from build123d import *

# Parameters (mm, degrees)
SKETCH_1_W              = 48
SKETCH_1_H              = 20
EXTRUDE_1_DEPTH         = 30
SKETCH_2_W              = 14
SKETCH_2_H              = 30
CUT_EXTRUDE_1_DEPTH     = 7
EXTRUDE_2_DEPTH         = 48
CUT_EXTRUDE_2_DEPTH     = 14
CUT_EXTRUDE_3_DEPTH     = 14
CUT_EXTRUDE_4_DEPTH     = 65.456478054
SKETCH_13_R             = 4
CUT_EXTRUDE_5_DEPTH     = 53.52066051
SKETCH_14_R             = 4
CUT_EXTRUDE_6_DEPTH     = 53.52066051
FILLET_1_R              = 7
EXTRUDE_3_DEPTH         = 3
EXTRUDE_5_DEPTH         = 1
SKETCH_20_R             = 7.5
CUT_EXTRUDE_8_DEPTH     = 53.520660579
BOSS_EXTRUDE1_DEPTH     = 25
CUT_EXTRUDE1_DEPTH      = 80.244164279
CUT_EXTRUDE1_DEPTH_BACK = 80.244164279


with BuildPart() as part:
    # Эскиз1 → Бобышка-Вытянуть1 (new body)
    with BuildSketch(Plane(origin=(0, 0, 0), x_dir=(1, 0, 0), z_dir=(0, 1, 0))):
        Rectangle(SKETCH_1_W, SKETCH_1_H)
    extrude(amount=EXTRUDE_1_DEPTH)

    # Эскиз2 → Вырез-Вытянуть1 (cut)
    with BuildSketch(Plane.XY.offset(10)):
        with Locations((0, 15)):
            Rectangle(SKETCH_2_W, SKETCH_2_H)
    extrude(amount=-CUT_EXTRUDE_1_DEPTH, mode=Mode.SUBTRACT)

    # Эскиз7 → Бобышка-Вытянуть2 (add)
    with BuildSketch(Plane(origin=(24, 0, 0), x_dir=(0, 0, -1), z_dir=(1, 0, 0))):
        Polygon((10, 0), (27.320508076, -10), (45.810889132, 22.026279442), (32, 30), (10, 30), align=None)
    extrude(amount=-EXTRUDE_2_DEPTH)

    # Эскиз8 → Вырез-Вытянуть2 (cut)
    with BuildSketch(Plane(origin=(24, 0, 0), x_dir=(0, 0, -1), z_dir=(1, 0, 0))):
        Polygon((10, 0), (10, 30), (32, 30), (45.810889132, 22.026279442), (27.320508076, -10), align=None)
    extrude(amount=-CUT_EXTRUDE_2_DEPTH, mode=Mode.SUBTRACT)

    # Эскиз9 → Вырез-Вытянуть3 (cut)
    with BuildSketch(Plane.ZY.offset(24)):
        Polygon((-10, 0), (-10, 30), (-32, 30), (-45.810889132, 22.026279442), (-27.320508076, -10), align=None)
    extrude(amount=-CUT_EXTRUDE_3_DEPTH, mode=Mode.SUBTRACT)

    # Эскиз11 → Вырез-Вытянуть4 (cut, through all)
    with BuildSketch(Plane.ZY.offset(10)):
        Polygon((-17.085266521, 5.482226936), (-27.285266521, 23.149145173), (-36.291930721, 17.949145173), (-26.091930721, 0.282226936), align=None)
    extrude(amount=-CUT_EXTRUDE_4_DEPTH, mode=Mode.SUBTRACT)

    # Эскиз13 → Вырез-Вытянуть5 (cut, through all)
    with BuildSketch(Plane(origin=(0, 0, -10), x_dir=(-1, 0, 0), z_dir=(0, 0, -1))):
        with Locations((17, 15)):
            Circle(SKETCH_13_R)
    extrude(amount=-CUT_EXTRUDE_5_DEPTH, mode=Mode.SUBTRACT)

    # Эскиз14 → Вырез-Вытянуть6 (cut, through all)
    with BuildSketch(Plane(origin=(0, 0, -10), x_dir=(-1, 0, 0), z_dir=(0, 0, -1))):
        with Locations((-17, 15)):
            Circle(SKETCH_14_R)
    extrude(amount=-CUT_EXTRUDE_6_DEPTH, mode=Mode.SUBTRACT)

    # Скругление1
    fillet_1_edges = [part.edges().sort_by_distance(p)[0] for p in [
        (-7, 15, 3),
        (7, 15, 3),
    ]]
    fillet(fillet_1_edges, radius=FILLET_1_R - 0.0001)  # a hair under: the kernel refuses the full size

    # Эскиз16 → Бобышка-Вытянуть3 (add)
    with BuildSketch(Plane(origin=(10, 0, 0), x_dir=(0, 0, -1), z_dir=(1, 0, 0))):
        Polygon((27.285266521, 23.149145173), (17.085266521, 5.482226936), (26.091930721, 0.282226936), (36.291930721, 17.949145173), align=None)
    extrude(amount=-EXTRUDE_3_DEPTH)

    # Эскиз18 → Бобышка-Вытянуть5 (add)
    with BuildSketch(Plane(origin=(0, -14.330127019, -24.820508076), x_dir=(-1, 0, 0), z_dir=(0, -0.4999999999999885, -0.8660254037844454))):
        with BuildLine():
            Line((3.076923077, 23.490381057), (3.076923077, 15.490381057))
            Line((3.076923077, 15.490381057), (-0.394230769, 15.490381057))
            add(Edge.make_bspline(
                [(-0.394230769, 15.490381057), (-0.475966203, 15.49101845), (-0.634155568, 15.49225205), (-0.863556464, 15.501067061), (-1.077173272, 15.519794557), (-1.276352297, 15.540710881), (-1.460752713, 15.571594241), (-1.630462401, 15.607825992), (-1.784830485, 15.650647709), (-1.925031539, 15.701264755), (-2.055118116, 15.758511595), (-2.175664232, 15.829183977), (-2.291845901, 15.906492451), (-2.399031866, 15.998074814), (-2.502049745, 16.096470161), (-2.596586483, 16.206601733), (-2.685439891, 16.325713037), (-2.793473896, 16.498197991), (-2.906939016, 16.729401784), (-3.004668447, 17.02314385), (-3.06681146, 17.330727068), (-3.073519576, 17.5408315), (-3.076923077, 17.647432339)],
                knots=[0, 0, 0, 0, 1.242075696, 2.40389213, 3.487198984, 4.500157661, 5.446319301, 6.326791195, 7.136300648, 7.878370406, 8.590488565, 9.292260633, 9.999224673, 10.708050372, 11.431369221, 12.162165018, 12.910600795, 13.687589445, 15.252257874, 16.810406251, 18.381693487, 20, 20, 20, 20], degree=3))
            add(Edge.make_bspline(
                [(-3.076923077, 17.647432339), (-3.075357604, 17.715865612), (-3.072265688, 17.851026019), (-3.048581646, 18.049748215), (-3.005726368, 18.239618444), (-2.950775925, 18.42230348), (-2.87555432, 18.595200652), (-2.788453183, 18.761894703), (-2.680395045, 18.917607923), (-2.559742342, 19.067544403), (-2.419445088, 19.204937793), (-2.263386964, 19.331922341), (-2.086876234, 19.440896432), (-1.89570213, 19.542168691), (-1.684937787, 19.625339579), (-1.457761732, 19.698574242), (-1.21241575, 19.755040234), (-1.042362796, 19.783482773), (-0.955128205, 19.798073364)],
                knots=[0, 0, 0, 0, 0.982645791, 1.940792824, 2.867691729, 3.775150443, 4.675643875, 5.571354211, 6.471357401, 7.392684514, 8.331098131, 9.285922955, 10.275520706, 11.304845665, 12.388884831, 13.524255008, 14.729980297, 16, 16, 16, 16], degree=3))
            add(Edge.make_bspline(
                [(-0.955128205, 19.798073364), (-1.019738399, 19.830278555), (-1.14226585, 19.891352818), (-1.308999482, 19.992404668), (-1.455065559, 20.087536339), (-1.53803712, 20.158871679), (-1.576923077, 20.192304134)],
                knots=[0, 0, 0, 0, 1.172551213, 2.223638478, 3.167479604, 4, 4, 4, 4], degree=3))
            add(Edge.make_bspline(
                [(-1.576923077, 20.192304134), (-1.652624383, 20.266285408), (-1.807875296, 20.418008818), (-2.019735444, 20.678834883), (-2.229368535, 20.965668904), (-2.355227865, 21.174690137), (-2.419871795, 21.282047723)],
                knots=[0, 0, 0, 0, 0.918170575, 1.883016652, 2.912673989, 4, 4, 4, 4], degree=3))
            Line((-2.419871795, 21.282047723), (-3.732371795, 23.490381057))
            Line((-3.732371795, 23.490381057), (-2.439102564, 23.490381057))
            Line((-2.439102564, 23.490381057), (-1.442307692, 21.801278493))
            add(Edge.make_bspline(
                [(-1.442307692, 21.801278493), (-1.406465761, 21.74201577), (-1.337009983, 21.627174345), (-1.236719552, 21.459429826), (-1.138255761, 21.30508177), (-1.047376022, 21.15932531), (-0.958316878, 21.02600434), (-0.878481314, 20.900073272), (-0.798305584, 20.788666158), (-0.706246053, 20.654823189), (-0.593818414, 20.510114732), (-0.462623309, 20.361457059), (-0.34199814, 20.238315643), (-0.18956943, 20.120822362), (-3.2323e-05, 20.013245791), (0.159774488, 19.962214344), (0.237179487, 19.937496441)],
                knots=[0, 0, 0, 0, 1.130591283, 2.190900266, 3.190104209, 4.119071823, 4.994606968, 5.807262858, 6.55236009, 7.234593472, 8.459046683, 9.540234366, 10.471327768, 11.266723835, 12.676093724, 14, 14, 14, 14], degree=3))
            add(Edge.make_bspline(
                [(0.237179487, 19.937496441), (0.269697183, 19.931632396), (0.343936058, 19.918244603), (0.469993483, 19.909501015), (0.622727518, 19.900220866), (0.733416476, 19.900491258), (0.793269231, 19.900637467)],
                knots=[0, 0, 0, 0, 0.709978628, 1.620902492, 2.713552433, 4, 4, 4, 4], degree=3))
            Line((0.793269231, 19.900637467), (1.948717949, 19.900637467))
            Line((1.948717949, 19.900637467), (1.948717949, 23.490381057))
            Line((1.948717949, 23.490381057), (3.076923077, 23.490381057))
        make_face()
        with BuildLine():
            Line((1.948717949, 18.977560544), (-0.193910256, 18.977560544))
            add(Edge.make_bspline(
                [(-0.193910256, 18.977560544), (-0.301354607, 18.97589409), (-0.502211742, 18.972778811), (-0.783007271, 18.945769758), (-1.023200158, 18.903550736), (-1.225858519, 18.839427155), (-1.396173113, 18.753553027), (-1.54378517, 18.648537277), (-1.667901131, 18.51825252), (-1.769975791, 18.368861713), (-1.849770319, 18.206056724), (-1.90552669, 18.03374763), (-1.942959563, 17.855238544), (-1.946787014, 17.733092852), (-1.948717949, 17.6714708)],
                knots=[0, 0, 0, 0, 1.546056516, 2.890207646, 4.055830773, 5.050253158, 5.937355789, 6.790906573, 7.644595853, 8.512568064, 9.38593768, 10.244184789, 11.114197691, 12, 12, 12, 12], degree=3))
            add(Edge.make_bspline(
                [(-1.948717949, 17.6714708), (-1.947235583, 17.626563151), (-1.944332064, 17.538602257), (-1.928948857, 17.409542216), (-1.89968097, 17.287236957), (-1.859266003, 17.17080484), (-1.808094758, 17.059993077), (-1.745213393, 16.955237495), (-1.670946372, 16.857073145), (-1.585753391, 16.765016757), (-1.487970747, 16.681241729), (-1.376270424, 16.608965458), (-1.251544399, 16.547545272), (-1.113644587, 16.498798364), (-0.963006292, 16.459808698), (-0.798771701, 16.43387015), (-0.621691971, 16.415101097), (-0.498985984, 16.414015918), (-0.435897436, 16.41345798)],
                knots=[0, 0, 0, 0, 0.965235723, 1.89061323, 2.787065514, 3.661873922, 4.534873316, 5.404925039, 6.281839248, 7.175200054, 8.095223355, 9.040740021, 10.02630299, 11.075573487, 12.177989335, 13.364883635, 14.645170704, 16, 16, 16, 16], degree=3))
            Line((-0.435897436, 16.41345798), (1.948717949, 16.41345798))
            Line((1.948717949, 16.41345798), (1.948717949, 18.977560544))
        make_face(mode=Mode.SUBTRACT)
    extrude(amount=EXTRUDE_5_DEPTH)

    # Эскиз20 → Вырез-Вытянуть8 (cut, through all)
    with BuildSketch(Plane(origin=(0, 0, -10), x_dir=(-1, 0, 0), z_dir=(0, 0, -1))):
        with Locations((-17, 15)):
            Circle(SKETCH_20_R)
        with Locations((17, 15)):
            Circle(SKETCH_20_R)
    extrude(amount=CUT_EXTRUDE_8_DEPTH, mode=Mode.SUBTRACT)

    # Sketch3 → Boss-Extrude1 (add)
    with BuildSketch(Plane(origin=(0, 30, 0), x_dir=(1, 0, 0), z_dir=(0, 1, 0))):
        with BuildLine():
            Line((7, -10), (24, -10))
            Line((24, -10), (24, 10))
            Line((24, 10), (10, 10))
            Line((10, 10), (10, 32))
            Line((10, 32), (-10, 32))
            Line((-10, 32), (-10, 10))
            Line((-10, 10), (-24, 10))
            Line((-24, 10), (-24, -10))
            Line((-24, -10), (-7, -10))
            ThreePointArc((-7, -10), (0, -3), (7, -10))
        make_face()
    extrude(amount=BOSS_EXTRUDE1_DEPTH)

    # Sketch4 → Cut-Extrude1 (cut, two sides: drawn at the far end of the back side and taken through both)
    with BuildSketch(Plane.ZY.offset(10).offset(-CUT_EXTRUDE1_DEPTH_BACK)):
        Polygon((-251.050138586, -96.468656479), (-45.810889132, 22.026279442), (35.63071017, 69.046608722), (240.869959624, 187.541544642), (3.880087783, 598.020043549), (-488.040010426, 314.009842428), align=None)
    extrude(amount=CUT_EXTRUDE1_DEPTH + CUT_EXTRUDE1_DEPTH_BACK, mode=Mode.SUBTRACT)


solid = part.part
Geometry check sheet. Reference: the model listing, model coordinates, mm. A direction names the side the tool comes from. Coordinates: 2 decimals unless noted, no trailing zeros. Order: outer loops, then holes, each group sorted by start corner. A loop starts at its lowest first (then second) coordinate and runs counter-clockwise, first axis right, second up. Notation, with made-up numbers: M 68.5,1 L 77.5,1 A33 ccw 77.5,37 Z; hole C -12.75,10.5 d9. An arc over 180 degrees is marked long. Use CSV: the item, a comma, the result in double quotes.
Item 1: Thickness scan on line 1 along Z through (x, y) = (-14, 39); line 2 along Y through (x, z) = (-3.5, -27.5). Record the ranges inside material, lowest first.
Returned:
line 1,"z = -10 to 10"
line 2,"y = -9.69 to 2.72, 23.03 to 32.6"
Item 2: Gauge pin test, flat ends, axial feed: pin 1 Ø7.5 at (y, z) = (26, -19) entering from +X; pin 2 Ø3 at (x, z) = (-1.5, -5) entering from +Y; pin 3 Ø10 at (x, z) = (16.5, 1.5) entering from -Y; pin 4 Ø5 at (x, y) = (-17, 15) entering from -Z. Record the tip position at first contact, or that the pin passes through.
Returned:
pin 1,"stops at x = 10"
pin 2,"stops at y = 46.45"
pin 3,"stops at y = 0"
pin 4,"passes through"
Item 3: Cross-section at D-D on z = 1. Record the cut outline in (x, y), then the cut area to 3 significant figures.
Returned:
outline,"M -24,0 L 24,0 L 24,49.05 L -24,49.05 Z; hole C -17,15 d8; hole C 17,15 d8"
area,"2,250 mm2"
Item 4: Tool access check on faces 1 (the flat face through (-1.619, 2.846, -21.652)), 2 (the flat face through (10, 27, -24)), 3 (the flat face through (3.067, 4.797, -36.433)), 4 (the flat face through (-3.077, 2, -35)), 5 (the flat face through (-10, 27, -24)). Record the directions out of +Z, -Z, +X, -X, +Y, -Y that give a thin tool (end or side, any length) a straight path to the whole face; none if there is none.
Returned:
face 1,"-X"
face 2,"-Z, +X, +Y, -Y"
face 3,"+X, -Y"
face 4,"-Z, -X, -Y"
face 5,"-Z, -X, +Y, -Y"
Item 5: Mould release check, pull along X, two halves, no side actions. Record for faces 6 (the flat face through (0.03, 0.98, -33.66)), 7 (the flat face through (-0.48, 2.1, -35.46)), 8 (the flat face through (24, 27, 0)): pulls with the +X half, pulls with the -X half, needs draft (parallel to the pull), parting line crosses it, or undercut.
Returned:
face 6,"undercut"
face 7,"needs draft"
face 8,"pulls with the +X half"
Item 6: Cross-section at B-B on x = -8. Record the cut outline in (y, z), then the cut area to 3 significant figures.
Returned:
outline,"M -10,-27.32 L 22.03,-45.81 L 54.25,10 L 0,10 L 0,-10 Z; hole M 0.28,-26.09 L 17.95,-36.29 L 23.15,-27.29 L 5.48,-17.09 Z"
area,"1,890 mm2"
Item 7: Cross-section at C-C on y = 15. Give the number of separate pieces and of enclosed holes in the cut face, then the cut area to 3 significant figures.
Returned:
separate pieces,"3"
enclosed holes,"0"
area,"968 mm2"
Item 8: Cross-section at A-A on x = 17. Record the cut outline in (y, z).
Returned:
outline,"M 0,-10 L 11,-10 L 11,10 L 0,10 Z; M 19,-10 L 42.7,-10 L 54.25,10 L 19,10 Z"
